The model under review builds one solid part; all positions refer to its coordinate system, in mm. A direction names the side the tool comes from. Give positions to 0.01 mm unless a question says otherwise; leave off trailing zeros. Order: outer loops, then holes, each group sorted by start corner. A loop starts at its lowest first (then second) coordinate and runs counter-clockwise, first axis right, second up. Notation, with made-up numbers: (2, 46.25) - (11, 46.25) arc R19 ccw to (11, 67.25) - close; hole circle Ø10 at (24.25, 71). An arc over 180 degrees is marked (long way). Write item = value, one per line. Start each with the question number.
1. We need section C-C, the plane y = 14.5. Give the boundary of the cut face in (x, z) (3 decimals), and give its area (3 significant figures).
2. Wall thickness on probe 1 along X at (y, z) = (-38.1, 5.5) (3 decimals); probe 2 along X at (y, z) = (0, 7); probe 3 along Y at (x, z) = (-101.6, 3.5) (3 decimals): over which ranges is each line inside the solid? List them lowest first.
3. For P1, Ø10, axis at x = -76.2, y = 38.1, coming from the -Z side; P2, Ø23, axis at x = 101.6, y = 0, coming from the -Z side; P3, Ø20, axis at x = -26, z = -38, coming from the -Y side; P4, Ø3, axis at x = -20, y = 70.5, coming from the -Z side (3 decimals), all flat-tipped, find the tip position at first contact; note any pin that passes through.
4. Mouldability with a two-part tool opening along X and no side actions: class faces 6 (the flat face through (127, 30, 2)), 7 (the flat face through (96, 68, -66.675)), 8 (the flat face through (1, 68, -28.575)) as pulls with the +X half, pulls with the -X half, needs draft (parallel to the pull), parting line crosses it, or undercut.
5. We need section A-A, the plane x = 76.2. Give the boundary of the cut face in (y, z) (3 decimals).
6. We need section B-B, the plane z = -34.5. Give the boundary of the cut face in (x, y) (3 decimals), and give its area (3 significant figures).
7. We need section D-D, the plane x = 23. Give the boundary of the cut face in (y, z) (3 decimals).
8. Machinability: for faces 1 (the flat face through (-2, 43, 0)), 2 (the flat face through (-1, -31.75, 5)), 3 (the flat face through (63.5, 68, -48)), 4 (the flat face through (2, 34, 9.525)), 5 (the flat face through (-2, -63.5, 5)), which of the approach directions +Z, -Z, +X, -X, +Y, -Y give a long, thin tool a straight path to every point of the face, cutting with its end or side? Answer none if there is none.
from build123d import *

# Parameters (mm, degrees)
F0_W     = 254
F0_H     = 127
F0_W_2   = 127
F0_H_2   = 63.5
F1_DEPTH = 9.525
F2_R     = 3.175
F3_DEPTH = 9525
F4_R     = 19.05
F5_DEPTH = 9.526
F6_W     = 254
F6_H     = 76.2
F7_DEPTH = 9.525
F8_W     = 127
F8_H     = 38.1
F9_DEPTH = 136.526


with BuildPart() as f1:
    # F0 (on Top) → F1 (new body)
    with BuildSketch(Plane.XY):
        Rectangle(F0_W, F0_H)
        Rectangle(F0_W_2, F0_H_2, mode=Mode.SUBTRACT)
    extrude(amount=F1_DEPTH)

    # F2 (on Top) → F3 (cut)
    with BuildSketch(Plane.XY):
        with Locations((-76.2, 38.1)):
            Circle(F2_R)
        with Locations((76.2, 38.1)):
            Circle(F2_R)
        with Locations((-76.2, -38.1)):
            Circle(F2_R)
        with Locations((76.2, -38.1)):
            Circle(F2_R)
    extrude(amount=F3_DEPTH, mode=Mode.SUBTRACT)

    # F4 (on Top) → F5 (cut, through all)
    with BuildSketch(Plane.XY):
        with Locations((-101.6, 0)):
            Circle(F4_R)
        with Locations((101.6, 0)):
            Circle(F4_R)
    extrude(amount=F5_DEPTH, mode=Mode.SUBTRACT)

    # F6 (on face) → F7 (join)
    with BuildSketch(Plane(origin=(0, 63.5, 0), x_dir=(-1, 0, 0), z_dir=(0, 1, 0))):
        with Locations((0, -28.575)):
            Rectangle(F6_W, F6_H)
    extrude(amount=F7_DEPTH)

    # F8 (on face) → F9 (cut, through all)
    with BuildSketch(Plane(origin=(0, 73.025, 0), x_dir=(-1, 0, 0), z_dir=(0, 1, 0))):
        with Locations((0, -47.625)):
            Rectangle(F8_W, F8_H)
    extrude(amount=-F9_DEPTH, mode=Mode.SUBTRACT)


solid = f1.part
Model answer:
q1.outline = (-127, 0) - (-113.955, 0) - (-113.955, 9.525) - (-127, 9.525) - close; (-89.245, 0) - (-63.5, 0) - (-63.5, 9.525) - (-89.245, 9.525) - close; (63.5, 0) - (89.245, 0) - (89.245, 9.525) - (63.5, 9.525) - close; (113.955, 0) - (127, 0) - (127, 9.525) - (113.955, 9.525) - close
q1.area = 739 mm2
q2.probe_1 = -127 to -79.375, -73.025 to 73.025, 79.375 to 127
q2.probe_2 = -127 to -120.65, -82.55 to -63.5, 63.5 to 82.55, 120.65 to 127
q2.probe_3 = -63.5 to -19.05, 19.05 to 73.025
q3.P1 = 0
q3.P2 = through
q3.P3 = 63.5
q3.P4 = -28.575
q4.face_6 = pulls with the +X half
q4.face_7 = needs draft
q4.face_8 = undercut
q5.outline = (-63.5, 0) - (-41.275, 0) - (-41.275, 9.525) - (-63.5, 9.525) - close; (-34.925, 0) - (34.925, 0) - (34.925, 9.525) - (-34.925, 9.525) - close; (41.275, 0) - (63.5, 0) - (63.5, -66.675) - (73.025, -66.675) - (73.025, 9.525) - (41.275, 9.525) - close
q6.outline = (-127, 63.5) - (-63.5, 63.5) - (-63.5, 73.025) - (-127, 73.025) - close; (63.5, 63.5) - (127, 63.5) - (127, 73.025) - (63.5, 73.025) - close
q6.area = 1,210 mm2
q7.outline = (-63.5, 0) - (-31.75, 0) - (-31.75, 9.525) - (-63.5, 9.525) - close; (31.75, 0) - (63.5, 0) - (63.5, -28.575) - (73.025, -28.575) - (73.025, 9.525) - (31.75, 9.525) - close
q8.face_1 = -Z, +X, -X, -Y
q8.face_2 = +Z, -Z
q8.face_3 = -Z, +Y, -Y
q8.face_4 = +Z, +X, -X, +Y, -Y
q8.face_5 = +Z, -Z, +X, -X, -Y
